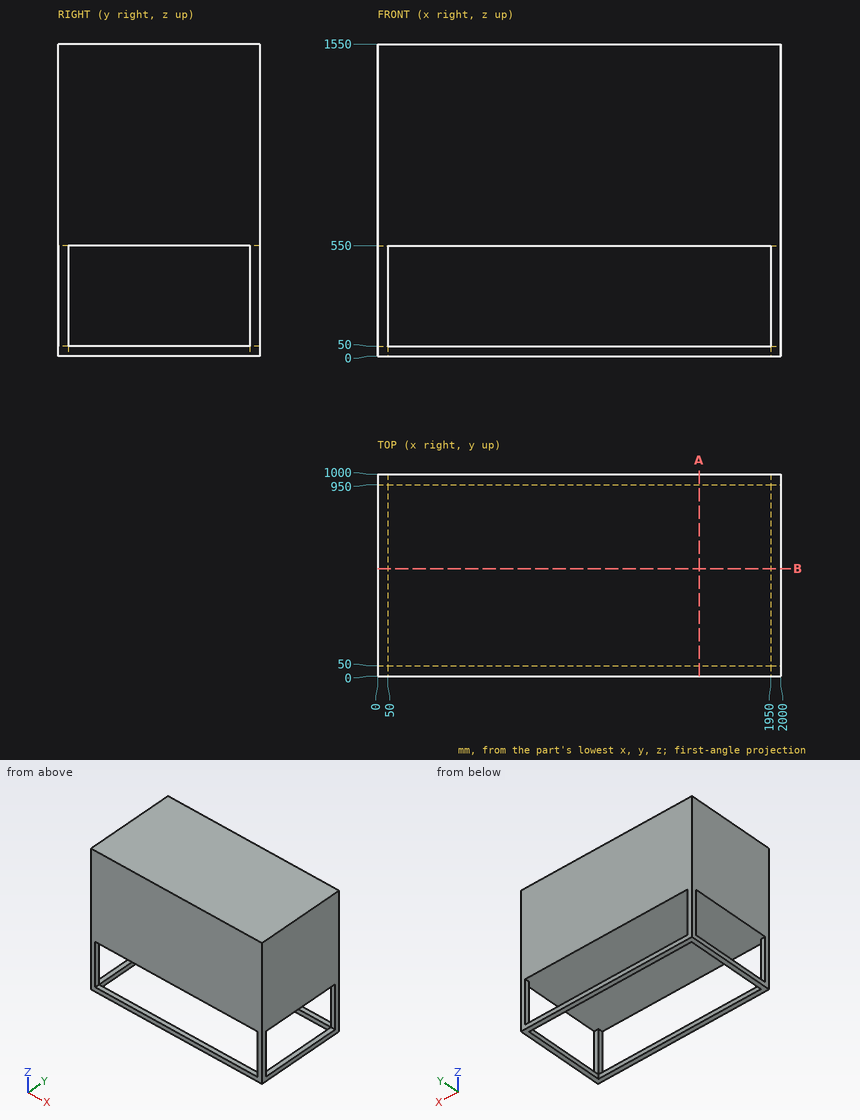
Study the drawing (mm; zero at the part's minimum x, y, z) and answer. Coordinates: 2 decimals unless noted, no trailing zeros. Loops run counter-clockwise (first coordinate to the right, second up) from the corner with the lowest first, then second, coordinate; pieces in that order, holes last. Notation, with made-up numbers: (14.25, -17) -> (21.25, -17) arc R17 ccw to (21.25, -3) -> close; hole circle Ø4 at (-39.75, 31). An arc over 180 degrees is marked (long way). Write item = value, one per line. Start each with the question number.
1) The part is cut by section A-A, the plane x = 1594. Determine the outline of the cut face in (y, z), plus the area to 4 significant figures.
2) The part is cut by section B-B, the plane y = 533. Determine the outline of the cut face in (x, z).
3) Given P1, Ø8, axis at x = 540.5, y = 559.5, coming from the -Z side; P2, Ø25, axis at y = 18.5, z = 182, coming from the -X side, each flat-ended and moving along its own axis, determine where each tip first touches the part or whether it passes through.
4) Find the intervals of material crossed by L1, parallel to Z at x = 529, y = 922.5, in increasing order. Write a range as from..to.
Result:
q1.outline = (0, 0) -> (50, 0) -> (50, 50) -> (0, 50) -> close; (0, 550) -> (1000, 550) -> (1000, 1550) -> (0, 1550) -> close; (950, 0) -> (1000, 0) -> (1000, 50) -> (950, 50) -> close
q1.area = 1,005,000 mm²
q2.outline = (0, 0) -> (50, 0) -> (50, 50) -> (0, 50) -> close; (0, 550) -> (2000, 550) -> (2000, 1550) -> (0, 1550) -> close; (1950, 0) -> (2000, 0) -> (2000, 50) -> (1950, 50) -> close
q3.P1 = 550
q3.P2 = 0
q4.L1 = 550..1550
